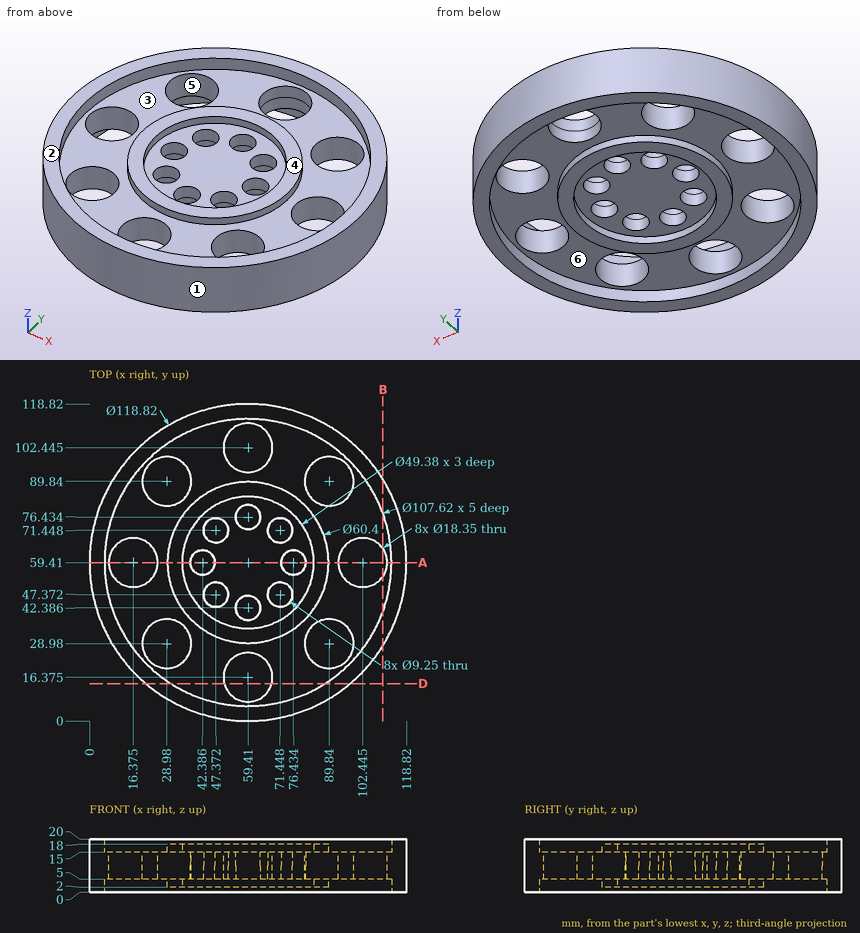
For this review, use the dimensioned drawing (mm, ordinates from the lowest corner) and the shaded views. A direction names the side the tool comes from. Round coordinates to 2 decimals unless told otherwise and drop trailing zeros. Write each loop counter-clockwise with the first axis right and the second up, starting at its lowest first coordinate (ties: lowest second). Pieces come first, ordered by that corner, then holes. Notation, with made-up numbers: M 74.25,63.25 L 102.25,63.25 A17 ccw 102.25,86.25 Z; hole C 19,20 d3. An arc over 180 degrees is marked long. Write item = value, one per line. Start each with the question number.
(1) The part is to be moulded in two halves that separate along Y. For the marked faces 1, 2 and 3, say which applies: +Y half, -Y half, draft (parallel to the pull), parting line (faces both ways), or undercut.
(2) For line 1 along Y through (x, z) = (59.41, 11.75); line 2 along Y through (x, z) = (59.41, 4.1), list the stretches that pass through material, from the lowest coordinate up.
(3) We need section B-B (x = 110). Give the boundary of the cut face in (y, z) (1 decimal).
(4) We need section D-D (y = 14). Give the boundary of the cut face in (x, z).
(5) We need section A-A (y = 59.41). Give the number of separate pieces and of enclosed holes in the cut face.
(6) For the marked faces 4, 5 and 6, list the 3-axis set-ups (+Z, -Z, +X, -X, +Y, -Y) from which the entire face can be reached by the end or side of a thin tool; tool diameter is ignored.
(7) Clearance check with flat-ended pins moving along their axes: pin 1 Ø5 at (y, z) = (34, 12.5) entering from +X (1 decimal); pin 2 Ø15 at (x, y) = (59.41, 42.39) entering from +Z; pin 3 Ø12 at (x, y) = (76.43, 59.41) entering from -Z. State where each tip first meets the part, or that it passes through.
Results found:
q1.face_1 = parting line
q1.face_2 = draft
q1.face_3 = undercut
q2.line_1 = 0 to 7.2, 25.55 to 37.76, 47.01 to 71.81, 81.06 to 93.27, 111.62 to 118.82
q2.line_2 = 0 to 5.6, 29.21 to 34.72, 84.1 to 89.61, 113.22 to 118.82
q3.outline = M 28.3,0 L 41.1,0 L 41.1,5 L 54.2,5 L 54.2,15 L 41.1,15 L 41.1,20 L 28.3,20 Z; M 64.6,5 L 77.7,5 L 77.7,0 L 90.6,0 L 90.6,20 L 77.7,20 L 77.7,15 L 64.6,15 Z
q4.outline = M 21.1,0 L 30.54,0 L 30.54,5 L 50.55,5 L 50.55,15 L 30.54,15 L 30.54,20 L 21.1,20 Z; M 68.27,5 L 88.28,5 L 88.28,0 L 97.72,0 L 97.72,20 L 88.28,20 L 88.28,15 L 68.27,15 Z
q5.separate_pieces = 5
q5.enclosed_holes = 0
q6.face_4 = +Z
q6.face_5 = +Z, -Z
q6.face_6 = -Z
q7.pin_1 = 114.2
q7.pin_2 = 15
q7.pin_3 = 5
